Read the model definition and answer for the solid it produces. Units are mm, in the model's axes. A direction names the side the tool comes from. Give positions to 0.01 mm unless a question says otherwise; leave off trailing zeros. Write each loop counter-clockwise with the first axis right and the second up, starting at its lowest first coordinate (ties: lowest second). Pieces come first, ordered by that corner, then holes. Notation, with made-up numbers: (49, 6) -> (69, 6) arc R25 cw to (69, 23) -> close; hole circle Ø3 at (-0.75, -15). An arc over 180 degrees is marked (long way). Use a Markdown table: item, result.
from build123d import *

# Parameters (mm, degrees)
SKETCH4_R           = 5
CUT_EXTRUDE4_DEPTH  = 16
BOSS_EXTRUDE1_DEPTH = 200
CIRPATTERN1_COUNT   = 5
SKETCH6_R           = 19.5
CUT_EXTRUDE5_DEPTH  = 291.086194087


with BuildPart() as part:
    # Sketch1 → Revolve2 (revolve)
    with BuildSketch(Plane.XY, mode=Mode.PRIVATE) as revolve2_sk:
        Polygon((-52.115384615, 0), (17.884615385, 0), (17.884615385, 75), (2.884615385, 75), (2.884615385, 70), (7.884615385, 70), (7.884615385, 20), (-42.115384615, 20), (-42.115384615, 70), (-37.115384615, 70), (-37.115384615, 75), (-52.115384615, 75), align=None)
    revolve(revolve2_sk.sketch.rotate(Axis((-114.1965821, 0, 0), (1, 0, 0)), 90), axis=Axis((-114.1965821, 0, 0), (1, 0, 0)))

    # Sketch4 → Cut-Extrude4 (cut)
    with BuildSketch(Plane(origin=(17.884615385, 0, 0), x_dir=(0, 0, -1), z_dir=(1, 0, 0))):
        with Locations((29.519700861, 0)):
            Circle(SKETCH4_R)
    extrude(amount=-CUT_EXTRUDE4_DEPTH, mode=Mode.SUBTRACT)

    # Sketch2 → Boss-Extrude1 (add)
    with BuildSketch(Plane.ZY.offset(52.115384615)):
        with BuildLine():
            Line((-18.650225291, 71.40454535), (-17.367191992, 65.951653826))
            ThreePointArc((-17.367191992, 65.951653826), (0, 68.2), (17.367191992, 65.951653826))
            Line((17.367191992, 65.951653826), (18.650225291, 71.40454535))
            ThreePointArc((18.650225291, 71.40454535), (0, 73.8), (-18.650225291, 71.40454535))
        make_face()
    boss_extrude1 = extrude(amount=BOSS_EXTRUDE1_DEPTH)

    # CirPattern1: Boss-Extrude1 ×5 about axis
    cirpattern1_axis = Axis((0, 0, 0), (1, 0, 0))
    for i in range(1, CIRPATTERN1_COUNT):
        add(boss_extrude1.rotate(cirpattern1_axis, i * 360 / CIRPATTERN1_COUNT))

    # Sketch6 → Cut-Extrude5 (cut, through all)
    with BuildSketch(Plane(origin=(17.884615385, 0, 0), x_dir=(0, 0, -1), z_dir=(1, 0, 0))):
        Circle(SKETCH6_R)
    extrude(amount=-CUT_EXTRUDE5_DEPTH, mode=Mode.SUBTRACT)


solid = part.part
Item 1: Straight lines are drawn through the part: line 1 along Y through (x, z) = (6, 0); line 2 along X through (y, z) = (-27.5, -33.5); line 3 along Y through (x, z) = (-27, 0). For each, find the intervals that lie inside material, in ascending order. Write a range as [from, to].
Return value:
| item | result |
|---|---|
| line 1 | [-75, -70], [-20, -19.5], [19.5, 20], [70, 75] |
| line 2 | [-52.12, -42.12], [7.88, 17.88] |
| line 3 | [-20, -19.5], [19.5, 20] |
Item 2: A cutting plane is placed at D-D (y = -34). Give the vertices of the cut face in (x, z), then the cut area to 3 significant figures.
Return value:
| item | result |
|---|---|
| outline | (-52.12, -66.85) -> (-37.12, -66.85) -> (-37.12, -61.19) -> (-42.12, -61.19) -> (-42.12, 61.19) -> (-37.12, 61.19) -> (-37.12, 66.85) -> (-52.12, 66.85) -> close; (2.88, -66.85) -> (17.88, -66.85) -> (17.88, 66.85) -> (2.88, 66.85) -> (2.88, 61.19) -> (7.88, 61.19) -> (7.88, -61.19) -> (2.88, -61.19) -> close |
| area | 2,790 mm^2 |
Item 3: A tool of negligible diameter and unlimited length cuts with its end or side. For faces 4 (the face through (-150.72, 4.1, -70.92)), 5 (the face through (5.42, 68.335, -15.175)), 6 (the face through (-150.715, -66.111, 25.783)), from which of +Z, -Z, +X, -X, +Y, -Y can it reach the whole face along a straight path? Write none if from no direction.
Return value:
| item | result |
|---|---|
| face 4 | -Z, -X, -Y |
| face 5 | none |
| face 6 | -X, -Y |
Item 4: A cutting plane is placed at A-A (y = 0). Give the vertices of the cut face in (x, z).
Return value:
| item | result |
|---|---|
| outline | (-52.12, -75) -> (-37.12, -75) -> (-37.12, -70) -> (-42.12, -70) -> (-42.12, -20) -> (7.88, -20) -> (7.88, -24.52) -> (17.88, -24.52) -> (17.88, -19.5) -> (-52.12, -19.5) -> close; (-52.12, 19.5) -> (17.88, 19.5) -> (17.88, 75) -> (2.88, 75) -> (2.88, 70) -> (7.88, 70) -> (7.88, 20) -> (-42.12, 20) -> (-42.12, 70) -> (-37.12, 70) -> (-37.12, 75) -> (-52.12, 75) -> close; (2.88, -75) -> (17.88, -75) -> (17.88, -34.52) -> (7.88, -34.52) -> (7.88, -70) -> (2.88, -70) -> close |
Item 5: A cutting plane is placed at B-B (x = -179). Give the vertices of the cut face in (y, z), then the cut area to 3 significant figures.
Return value:
| item | result |
|---|---|
| outline | (-68.73, -26.88) arc R73.8 ccw to (-46.81, -57.06) -> (-43.15, -52.82) arc R68.2 cw to (-63.56, -24.72) -> close; (-68.73, 26.88) -> (-63.56, 24.72) arc R68.2 cw to (-43.15, 52.82) -> (-46.81, 57.06) arc R73.8 ccw to start; (3.86, -68.09) -> (4.33, -73.67) arc R73.8 ccw to (39.8, -62.15) -> (36.9, -57.36) arc R68.2 cw to start; (3.86, 68.09) arc R68.2 cw to (36.9, 57.36) -> (39.8, 62.15) arc R73.8 ccw to (4.33, 73.67) -> close; (65.95, -17.37) -> (71.4, -18.65) arc R73.8 ccw to (71.4, 18.65) -> (65.95, 17.37) arc R68.2 cw to start |
| area | 1,020 mm^2 |
Item 6: A cutting plane is placed at C-C (z = 0). Give the vertices of the cut face in (x, y).
Return value:
| item | result |
|---|---|
| outline | (-252.12, 68.2) -> (-52.12, 68.2) -> (-52.12, 19.5) -> (17.88, 19.5) -> (17.88, 75) -> (2.88, 75) -> (2.88, 70) -> (7.88, 70) -> (7.88, 20) -> (-42.12, 20) -> (-42.12, 70) -> (-37.12, 70) -> (-37.12, 75) -> (-52.12, 75) -> (-52.12, 73.8) -> (-252.12, 73.8) -> close; (-52.12, -75) -> (-37.12, -75) -> (-37.12, -70) -> (-42.12, -70) -> (-42.12, -20) -> (7.88, -20) -> (7.88, -70) -> (2.88, -70) -> (2.88, -75) -> (17.88, -75) -> (17.88, -19.5) -> (-52.12, -19.5) -> close |
Item 7: For a pull along X with two mould halves and no side action, classify faces 1 (the face through (-52.115, 16, 16)), 2 (the face through (-39.58, 68.335, -15.175)), 3 (the face through (10.28, 66.538, 34.608)) as +X half, -X half, draft (parallel to the pull), parting line (faces both ways), or undercut.
Return value:
| item | result |
|---|---|
| face 1 | -X half |
| face 2 | undercut |
| face 3 | draft |
Item 8: Each of these flat-tipped pins is pushed along its axis until it touches: P1, Ø6, axis at x = -53.5, z = -0.5, coming from the -Y side; P2, Ø8, axis at x = -155, z = -55.5, coming from the +Y side; P3, Ø10, axis at x = -192.5, z = -5.5, coming from the +Y side. Where does it stop, or does it pass through?
Return value:
| item | result |
|---|---|
| P1 | y = -75 |
| P2 | y = 38.2 |
| P3 | y = 73.8 |
